```python
from build123d import *

# Parameters (mm, degrees)
PAD_DEPTH       = 75
POCKET_DEPTH    = 73
SKETCH002_R     = 1.25
SKETCH002_W     = 30
SKETCH002_H     = 60
POCKET001_DEPTH = 5
SKETCH005_W     = 10
SKETCH005_H     = 20
POCKET002_DEPTH = 2
SKETCH004_W     = 15
SKETCH004_H     = 15
POCKET003_DEPTH = 5
POCKET004_DEPTH = 1.5


with BuildPart() as part:
    # Sketch → Pad (new body)
    with BuildSketch(Plane.XY):
        Polygon((-15, 28.7253277197), (-15, -6.2746722803), (5, -20.9156884317), (20, -20.9156884317), (20, -5.9156884317), (0, 28.7253277197), align=None)
    extrude(amount=PAD_DEPTH)

    # Sketch001 (on Face7 of Pad) → Pocket (cut)
    with BuildSketch(Plane(origin=(0, 0, 0), x_dir=(1, 0, 0), z_dir=(0, 0, -1))):
        Polygon((-13, 4.2746722803), (7, 18.9156884317), (18, 18.9156884317), (18, 6.4515868166), (-1.1547005384, -26.7253277197), (-13, -26.7253277197), align=None)
    extrude(amount=-POCKET_DEPTH, mode=Mode.SUBTRACT)

    # Sketch002 (on Face6 of Pocket) → Pocket001 (cut)
    with BuildSketch(Plane(origin=(12.4384317686, 7.1813319299, 0), x_dir=(-0.5, 0.8660254038, 0), z_dir=(0.8660254038, 0.5, 0))):
        with Locations((-11.8731364627, 69)):
            Circle(SKETCH002_R)
        with Locations((21.6268635373, 6.75)):
            Circle(SKETCH002_R)
        with Locations((-11.8731364627, 6.75)):
            Circle(SKETCH002_R)
        with Locations((21.6268635373, 69)):
            Circle(SKETCH002_R)
        with Locations((4.8768635373, 35)):
            Rectangle(SKETCH002_W, SKETCH002_H)
    extrude(amount=-POCKET001_DEPTH, mode=Mode.SUBTRACT)

    # Sketch005 (on Face2 of Pocket001) → Pocket002 (cut)
    with BuildSketch(Plane(origin=(0, 28.7253277197, 0), x_dir=(-1, 0, 0), z_dir=(0, 1, 0))):
        with Locations((4, 56)):
            Rectangle(SKETCH005_W, SKETCH005_H)
    extrude(amount=-POCKET002_DEPTH, mode=Mode.SUBTRACT)

    # Sketch004 (on Face8 of Pocket001) → Pocket003 (cut)
    with BuildSketch(Plane.YZ.offset(20)):
        with Locations((-13.4156884317, 47.5)):
            Rectangle(SKETCH004_W, SKETCH004_H)
    extrude(amount=-POCKET003_DEPTH, mode=Mode.SUBTRACT)

    # Sketch006 (on Face12 of Pocket003) → Pocket004 (cut)
    with BuildSketch(Plane(origin=(-6.5733230776, -8.9793263113, 0), x_dir=(-0.8068982214, 0.5906904946, 0), z_dir=(0.5906904946, 0.8068982214, 0))):
        with BuildLine():
            ThreePointArc((7.2285743414, 50.5731403336), (-4.2714256586, 62.0731403336), (-15.7714256586, 50.5731403336))
            Line((-15.7714256586, 50.5731403336), (-15.7714256586, 23.5731403336))
            ThreePointArc((-15.7714256586, 23.5731403336), (-4.2714256586, 12.0731403336), (7.2285743414, 23.5731403336))
            Line((7.2285743414, 50.5731403336), (7.2285743414, 23.5731403336))
        make_face()
    extrude(amount=-POCKET004_DEPTH, mode=Mode.SUBTRACT)


solid = part.part
```
The listing builds one solid part. Answer for the finished solid, in the listing's coordinates (mm). A direction names the side the tool comes from. Give positions to 0.01 mm unless a question says otherwise; leave off trailing zeros. Write each loop counter-clockwise with the first axis right and the second up, starting at its lowest first coordinate (ties: lowest second). Pieces come first, ordered by that corner, then holes. Notation, with made-up numbers: (57, 32) - (98, 32) arc R21 ccw to (98, 69) - close; hole circle Ø8 at (34, -33). An arc over 180 degrees is marked (long way). Use one line per item in the form item = value. Start each with the question number.
1) Consider line 1 along X through (y, z) = (8.5, 51); line 2 along Z through (x, y) = (-3.5, -4); line 3 along Y through (x, z) = (10.5, 36). Determine where each line is inside the solid, lowest interval first. Write a range as from..to.
2) Find section D-D on x = 12.5. Determine the outline of the cut face in (y, z), plus the area to 3 significant figures.
3) Find section B-B on y = 5. Determine the outline of the cut face in (x, z).
4) Find section A-A on z = 44. Determine the outline of the cut face in (x, y), plus the area to 3 significant figures.
5) Find section C-C on z = 10. Determine the outline of the cut face in (x, y).
6) Flat-ended cylindrical pins translate along their axes: pin 1 Ø2 at (x, y) = (6.5, 11) entering from -Z; pin 2 Ø13 at (x, z) = (-7.5, 40.5) entering from -Y; pin 3 Ø2 at (y, z) = (-20.5, 49) entering from +X. Find the tip coordinate at first contact, or state that the pin passes through.
7) The mould has two halves that part along Y. Classify faces 1 (the face through (3, 4, 73)), 2 (the face through (19, -14, 40)), 3 (the face through (12, -20.916, 37)): pulls with the +Y half, pulls with the -Y half, needs draft (parallel to the pull), parting line crosses it, or undercut.
8) A tool of negligible diameter and unlimited length cuts with its end or side. For faces 4 (the face through (18, -13, 64)), 5 (the face through (0, 26.725, 56)), 6 (the face through (19, -14, 55)), 7 (the face through (1.646, 23.902, 34.58)), from which of +Z, -Z, +X, -X, +Y, -Y can it reach the whole face along a straight path? Write none if from no direction.
Geometry results:
q1.line_1 = -15..-13
q1.line_2 = 73..75
q1.line_3 = -20.92..-18.92
q2.outline = (-20.92, 0) - (-18.92, 0) - (-18.92, 73) - (3.07, 73) - (3.07, 65) - (7.07, 65) - (7.07, 75) - (-20.92, 75) - close; (3.07, 0) - (7.07, 0) - (7.07, 5) - (3.07, 5) - close
q2.area = 254 mm2
q3.outline = (-15, 0) - (-13, 0) - (-13, 73) - (11.39, 73) - (11.39, 65) - (13.7, 65) - (13.7, 75) - (-15, 75) - close; (11.39, 0) - (13.7, 0) - (13.7, 5) - (11.39, 5) - close
q4.outline = (-15, -6.27) - (5, -20.92) - (15, -20.92) - (15, -18.92) - (7, -18.92) - (6.15, -18.3) - (5.27, -19.51) - (-13.29, -5.92) - (-12.41, -4.71) - (-13, -4.27) - (-13, 26.73) - (-1.15, 26.73) - (0.77, 23.4) - (2.5, 24.4) - (0, 28.73) - (-15, 28.73) - close; (15.77, -2.59) - (17.69, -5.92) - (20, -5.92) - (17.5, -1.59) - close
q4.area = 163 mm2
q5.outline = (-15, -6.27) - (5, -20.92) - (20, -20.92) - (20, -5.92) - (17.5, -1.59) - (15.77, -2.59) - (18, -6.45) - (18, -18.92) - (7, -18.92) - (-13, -4.27) - (-13, 26.73) - (-1.15, 26.73) - (0.77, 23.4) - (2.5, 24.4) - (0, 28.73) - (-15, 28.73) - close
q6.pin_1 = 73
q6.pin_2 = -16.52
q6.pin_3 = 15
q7.face_1 = undercut
q7.face_2 = needs draft
q7.face_3 = pulls with the -Y half
q8.face_4 = -Z
q8.face_5 = +Y
q8.face_6 = +X, -Y
q8.face_7 = +X
